```python
from build123d import *

# Parameters (mm, degrees)
SKETCH016_W  = 70
SKETCH016_H  = 70
SKETCH016_R  = 1.6
PAD012_DEPTH = 5
PAD013_DEPTH = 12
SKETCH018_W  = 35
SKETCH018_H  = 35
PAD014_DEPTH = 7.5


with BuildPart() as part:
    # Sketch016 → Pad012 (new body)
    with BuildSketch(Plane.XZ):
        Rectangle(SKETCH016_W, SKETCH016_H)
        with Locations((-30, -24)):
            Circle(SKETCH016_R, mode=Mode.SUBTRACT)
        with Locations((-11, 31)):
            Circle(SKETCH016_R, mode=Mode.SUBTRACT)
    extrude(amount=-PAD012_DEPTH)

    # Sketch017 (on Face8 of Pad012) → Pad013 (join)
    with BuildSketch(Plane(origin=(0, 5, 0), x_dir=(1, 0, 0), z_dir=(0, 1, 0))):
        Polygon((-20, 27), (-33, 14), (-33, -8), (-20, -8), (-6, -32), (33, -32), (33, 21), (27, 21), (27, 27), align=None)
    extrude(amount=PAD013_DEPTH)

    # Sketch018 (on Face18 of Pad013) → Pad014 (join)
    with BuildSketch(Plane(origin=(0, 17, 0), x_dir=(1, 0, 0), z_dir=(0, 1, 0))):
        with Locations((13, -12.5)):
            Rectangle(SKETCH018_W, SKETCH018_H)
    extrude(amount=PAD014_DEPTH)


with BuildPart() as part_1:
    # Body010 placement: moved
    add(part.part.moved(Location((0, 16.5, -80.2))))


solid = part_1.part
```
The model under review builds one solid part; all positions refer to its coordinate system, in mm. A direction names the side the tool comes from. Give positions to 0.01 mm unless a question says otherwise; leave off trailing zeros. Write each loop counter-clockwise with the first axis right and the second up, starting at its lowest first coordinate (ties: lowest second). Pieces come first, ordered by that corner, then holes.
(1) Consider section A-A, the plane z = -104.2. Give the boundary of the cut face in (x, y).
(2) The part is to be moulded in two halves that separate along X. For faces 4 (the flat face through (-27, 27, -72.2)), 5 (the cylindrical face through (-12.27, 18.96, -50.17)), 6 (the flat face through (-13.1, 27.42, -60.37)), say which applies: released by +X, released by -X, zero draft, split by the parting line, or undercut.
(3) Tool access review of faces 1 (the flat face through (4, 27, -107.2)), 2 (the flat face through (30, 27, -101.2)), 3 (the flat face through (33, 27, -74)): name each direction out of +Z, -Z, +X, -X, +Y, -Y from which nothing blocks a thin tool from reaching the whole face with its end or side.
(4) Consider section C-C, the plane x = 14. Give the boundary of the cut face in (y, z).
(5) Consider section B-B, the plane y = 28.75. Give the boundary of the cut face in (x, z).
(6) Consider section D-D, the plane x = -11. Give the boundary of the cut face in (y, z), and give its area (3 significant figures).
(7) For P1, Ø2, axis at y = 39, z = -74, coming from the +X side; P2, Ø10, axis at x = -4.5, y = 33.5, coming from the +Z side; P3, Ø6, axis at y = 30, z = -72, coming from the -X side, all flat-tipped, find the tip position at first contact; note any pin that passes through.
(8) To check wall thickness, follow L1, parallel to X at y = 19.5, z = -104.2; L2, parallel to Y at x = 8, z = -104; L3, parallel to Y at x = -17.5, z = -55. State the ranges of each line that lie inside material, in increasing order.
Returned:
1. outline: (-35, 16.5) - (-31.6, 16.5) - (-31.6, 21.5) - (-35, 21.5) - close; (-28.4, 16.5) - (35, 16.5) - (35, 21.5) - (27, 21.5) - (27, 33.5) - (-23, 33.5) - (-23, 21.5) - (-28.4, 21.5) - close
2. face 4: zero draft
2. face 5: undercut
2. face 6: released by -X
3. face 1: -Z, +X, -X, +Y
3. face 2: -Z, +X, +Y
3. face 3: +Z, -Z, +X, +Y
4. outline: (16.5, -115.2) - (21.5, -115.2) - (21.5, -107.2) - (33.5, -107.2) - (33.5, -85.2) - (41, -85.2) - (41, -50.2) - (33.5, -50.2) - (33.5, -48.2) - (21.5, -48.2) - (21.5, -45.2) - (16.5, -45.2) - close
5. outline: (-33, -94.2) - (-20, -107.2) - (27, -107.2) - (27, -101.2) - (33, -101.2) - (33, -48.2) - (-6, -48.2) - (-20, -72.2) - (-33, -72.2) - close
6. outline: (16.5, -115.2) - (21.5, -115.2) - (21.5, -107.2) - (33.5, -107.2) - (33.5, -56.77) - (21.5, -56.77) - (21.5, -50.8) - (16.5, -50.8) - close; (16.5, -47.6) - (21.5, -47.6) - (21.5, -45.2) - (16.5, -45.2) - close
6. area: 939 mm2
7. P1: stops at x = 30.5
7. P2: stops at z = -48.2
7. P3: stops at x = -33
8. L1: x = -35 to -31.6, -28.4 to 35
8. L2: y = 16.5 to 33.5
8. L3: y = 16.5 to 21.5
